Geometry: final body of the model. Coordinates: model frame, mm. A direction names the side the tool comes from. Give positions to 0.01 mm unless a question says otherwise; leave off trailing zeros. Write each loop counter-clockwise with the first axis right and the second up, starting at its lowest first coordinate (ties: lowest second). Pieces come first, ordered by that corner, then holes.
```python
from build123d import *

# Parameters (mm, degrees)
SKETCH1_R           = 37.843146067
BOSS_EXTRUDE1_DEPTH = 12.7
SKETCH2_R           = 3.759495298
BOSS_EXTRUDE2_DEPTH = 5.08
SKETCH4_R           = 4.642939976
CUT_EXTRUDE1_DEPTH  = 56.00452171
CIRPATTERN1_COUNT   = 8


with BuildPart() as part:
    # Sketch1 → Boss-Extrude1 (new body)
    with BuildSketch(Plane.XY):
        Circle(SKETCH1_R)
    extrude(amount=BOSS_EXTRUDE1_DEPTH)

    # Sketch2 → Boss-Extrude2 (add)
    with BuildSketch(Plane.XY.offset(12.7)):
        Circle(SKETCH2_R)
    extrude(amount=BOSS_EXTRUDE2_DEPTH)

    # Sketch4 → Cut-Extrude1 (cut, through all)
    with BuildSketch(Plane.XY.offset(12.7)):
        with Locations((27.688174832, 0)):
            Circle(SKETCH4_R)
    cut_extrude1 = extrude(amount=-CUT_EXTRUDE1_DEPTH, mode=Mode.SUBTRACT)

    # CirPattern1: Cut-Extrude1 ×8 about axis
    cirpattern1_axis = Axis((0, 0, 0), (0, 0, 1))
    for i in range(1, CIRPATTERN1_COUNT):
        add(cut_extrude1.rotate(cirpattern1_axis, i * 360 / CIRPATTERN1_COUNT), mode=Mode.SUBTRACT)


solid = part.part
```
Item 1: Pin query (flat end, axial travel): pin 1 Ø6 at (x, y) = (-10, 13.5) entering from +Z; pin 2 Ø6 at (y, z) = (-8.5, 4) entering from -X; pin 3 Ø1.5 at (y, z) = (-13, 11) entering from -X; pin 4 Ø10.5 at (x, y) = (19.58, -19.58) entering from -Z. Return the tip coordinate at first contact, or that it passes through.
Found:
pin 1: stops at z = 12.7
pin 2: stops at x = -37.44
pin 3: stops at x = -35.81
pin 4: stops at z = 0
Item 2: Pull-direction query (X, two-part tool) for faces 3 (the face through (-15.9, -22.41, 6.44)), 4 (the face through (22.41, -15.9, 6.44)), 5 (the face through (-1, 1, 0)), 6 (the face through (-8.204, -36.943, 6.261)); classes: +X half, -X half, draft (parallel to the pull), parting line (faces both ways), or undercut.
Found:
face 3: undercut
face 4: undercut
face 5: draft
face 6: parting line
Item 3: Reachability of faces 1 (the face through (23.05, 0.2, 6.44)), 2 (the face through (3.586, 1.129, 15.204)) from +Z, -Z, +X, -X, +Y, -Y: full face, straight path, thin tool, end or side. Return the list, or none.
Found:
face 1: +Z, -Z
face 2: +Z
Item 4: Section A-A, the plane y = 0. Return the cut outline in (x, z).
Found:
outline: (-37.84, 0) - (-32.33, 0) - (-32.33, 12.7) - (-37.84, 12.7) - close; (-23.05, 0) - (23.05, 0) - (23.05, 12.7) - (3.76, 12.7) - (3.76, 17.78) - (-3.76, 17.78) - (-3.76, 12.7) - (-23.05, 12.7) - close; (32.33, 0) - (37.84, 0) - (37.84, 12.7) - (32.33, 12.7) - close
Item 5: Line query: L1, parallel to Y at x = 20.5, z = 3.25; L2, parallel to X at y = 3, z = 10.75; L3, parallel to X at y = 18.5, z = 10.25. Output: solid intervals per line, ascending.
Found:
L1: y = -31.81 to -24.13, -15.03 to 15.03, 24.13 to 31.81
L2: x = -37.72 to -31.23, -24.14 to 24.14, 31.23 to 37.72
L3: x = -33.01 to -24.09, -15.06 to 15.06, 24.09 to 33.01
Item 6: Section C-C, the plane z = 7.5. State how many separate pieces and enclosed holes the cut face has, plus the area to 3 significant figures.
Found:
separate pieces: 1
enclosed holes: 8
area: 3,960 mm2
Item 7: Section D-D, the plane y = 20. Return the cut outline in (x, z), plus the area to 3 significant figures.
Found:
outline: (-32.13, 0) - (-24.2, 0) - (-24.2, 12.7) - (-32.13, 12.7) - close; (-14.95, 0) - (14.95, 0) - (14.95, 12.7) - (-14.95, 12.7) - close; (24.2, 0) - (32.13, 0) - (32.13, 12.7) - (24.2, 12.7) - close
area: 581 mm2
